Source: three-view drawing plus pictorial views. Frame: mm from the lowest corner of the part. A direction names the side the tool comes from. Coordinates: 2 decimals unless noted, no trailing zeros. Loops run counter-clockwise (first coordinate to the right, second up) from the corner with the lowest first, then second, coordinate; pieces in that order, holes last. Notation, with made-up numbers: (-8.75, -38) - (36.25, -38) arc R18 ccw to (36.25, -10) - close; hole circle Ø7 at (52, -28). An arc over 180 degrees is marked (long way). Return JSON: item names as keys, results as strings.
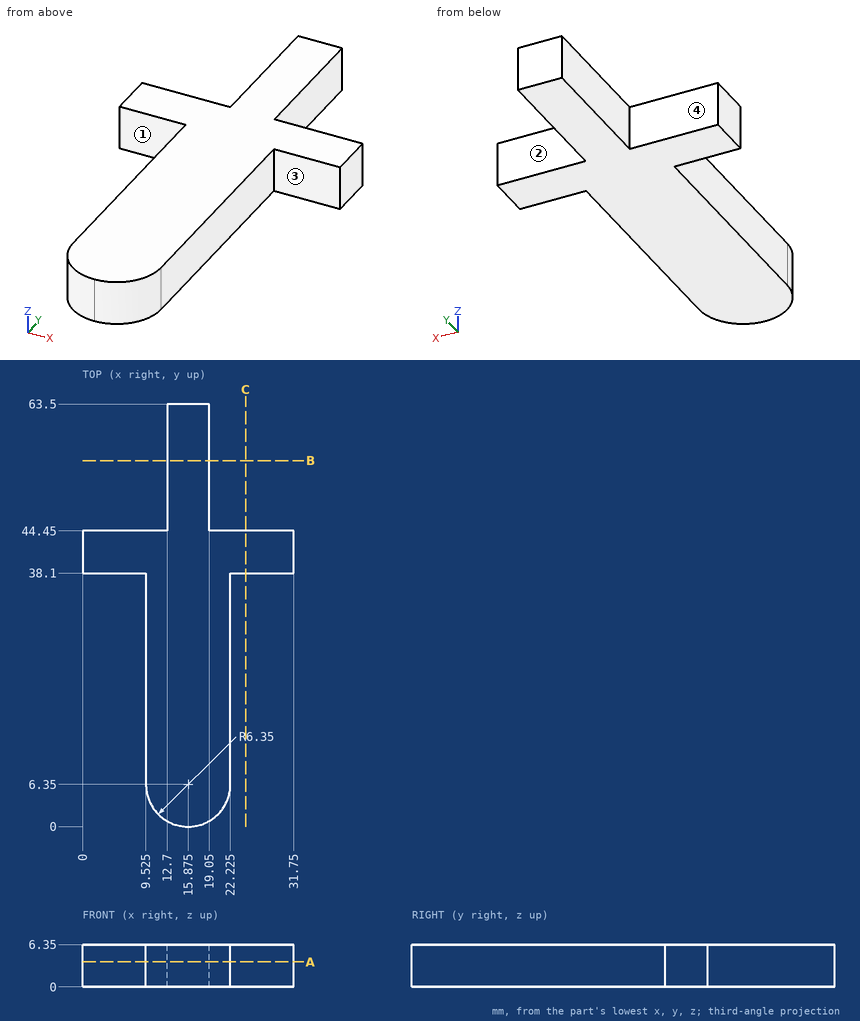
Item 1: First-contact query: pin 1 Ø3 at (x, z) = (27.5, 1.5) entering from +Y; pin 2 Ø3 at (y, z) = (27, 3) entering from -X (3 decimals); pin 3 Ø6 at (x, y) = (24, 47.5) entering from -Z; pin 4 Ø1.9 at (x, z) = (5.5, 2.5) entering from -Y. Flat tips, straight axial feed; report the tip coordinate or a pass-through.
Worked out:
{"pin 1": "y = 44.45", "pin 2": "x = 9.525", "pin 3": "through", "pin 4": "y = 38.1"}
Item 2: Ray query, probe 1 along X at (y, z) = (17, 4) (3 decimals); probe 2 along Y at (x, z) = (22.5, 2.5); probe 3 along X at (y, z) = (50.5, 4.5). Return the intervals inside material, ascending. Write a range as from..to.
Worked out:
{"probe 1": "9.525..22.225", "probe 2": "38.1..44.45", "probe 3": "12.7..19.05"}
Item 3: Section query C-C, the plane x = 24.5. Return loops of the section in (y, z), and give its area (3 significant figures).
Worked out:
{"outline": "(38.1, 0) - (44.45, 0) - (44.45, 6.35) - (38.1, 6.35) - close", "area": "40.3 mm^2"}
Item 4: Section query A-A, the plane z = 3.75. Return loops of the section in (x, y) (3 decimals).
Worked out:
{"outline": "(0, 38.1) - (9.525, 38.1) - (9.525, 6.35) arc R6.35 ccw to (22.225, 6.35) - (22.225, 38.1) - (31.75, 38.1) - (31.75, 44.45) - (19.05, 44.45) - (19.05, 63.5) - (12.7, 63.5) - (12.7, 44.45) - (0, 44.45) - close"}
Item 5: Reachability of the marked faces 1, 2, 3 and 4 from +Z, -Z, +X, -X, +Y, -Y: full face, straight path, thin tool, end or side. Return the list, or none.
Worked out:
{"face 1": "+Z, -Z, -X, -Y", "face 2": "+Z, -Z, +X, +Y", "face 3": "+Z, -Z, +X, -Y", "face 4": "+Z, -Z, -X, +Y"}
Item 6: Section query B-B, the plane y = 55. Return loops of the section in (x, z), and give its area (3 significant figures).
Worked out:
{"outline": "(12.7, 0) - (19.05, 0) - (19.05, 6.35) - (12.7, 6.35) - close", "area": "40.3 mm^2"}
